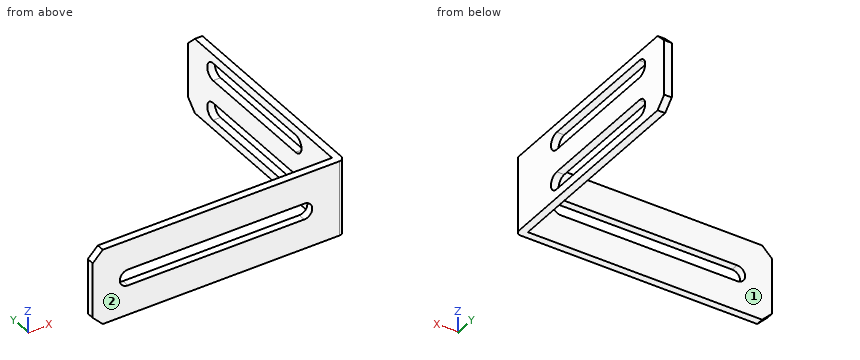
from build123d import *

# Parameters (mm, degrees)
BOSS_EXTRUDE1_DEPTH = 15
CUT_EXTRUDE1_DEPTH  = 2.5
CUT_EXTRUDE2_DEPTH  = 2.5
CHAMFER1_SIZE       = 2
FILLET1_R           = 1


with BuildPart() as part:
    # Sketch1 → Boss-Extrude1 (new body)
    with BuildSketch(Plane.XY):
        Polygon((-218.84057971, 0), (-170.34057971, 0), (-170.34057971, 43.5), (-168.84057971, 43.5), (-168.84057971, -1.5), (-218.84057971, -1.5), align=None)
    extrude(amount=BOSS_EXTRUDE1_DEPTH)

    # Sketch2 → Cut-Extrude1 (cut, through all)
    with BuildSketch(Plane(origin=(0, 0, 0), x_dir=(1, 0, 0), z_dir=(0, 1, 0))):
        with BuildLine():
            Line((-176.854809789, -9.1), (-211.854809789, -9.1))
            ThreePointArc((-211.854809789, -9.1), (-213.454809789, -7.5), (-211.854809789, -5.9))
            Line((-211.854809789, -5.9), (-176.854809789, -5.9))
            ThreePointArc((-176.854809789, -5.9), (-175.254809789, -7.5), (-176.854809789, -9.1))
        make_face()
    extrude(amount=-CUT_EXTRUDE1_DEPTH, mode=Mode.SUBTRACT)

    # Sketch3 → Cut-Extrude2 (cut, through all)
    with BuildSketch(Plane.ZY.offset(170.34057971)):
        with BuildLine():
            Line((1.75, 36), (1.75, 11))
            ThreePointArc((1.75, 11), (3.5, 9.25), (5.25, 11))
            Line((5.25, 11), (5.25, 36))
            ThreePointArc((5.25, 36), (3.5, 37.75), (1.75, 36))
        make_face()
        with BuildLine():
            Line((9.75, 36), (9.75, 11))
            ThreePointArc((9.75, 11), (11.5, 9.25), (13.25, 11))
            Line((13.25, 11), (13.25, 36))
            ThreePointArc((13.25, 36), (11.5, 37.75), (9.75, 36))
        make_face()
    extrude(amount=-CUT_EXTRUDE2_DEPTH, mode=Mode.SUBTRACT)

    # Chamfer1
    chamfer1_edges = [part.edges().sort_by_distance(p)[0] for p in [
        (-169.59057971, 43.5, 15),
        (-218.84057971, -0.75, 15),
        (-169.59057971, 43.5, 0),
        (-218.84057971, -0.75, 0),
    ]]
    chamfer(chamfer1_edges, length=CHAMFER1_SIZE)

    # Fillet1
    fillet1_edges = [part.edges().sort_by_distance(p)[0] for p in [
        (-168.84057971, -1.5, 7.5),
    ]]
    fillet(fillet1_edges, radius=FILLET1_R)


solid = part.part
Input: part model. Units: mm. Frame: model coordinates. Face numbers are marked on the shaded views. A direction names the side the tool comes from. Coordinates: 2 decimals unless noted, no trailing zeros. Loops run counter-clockwise (first coordinate to the right, second up) from the corner with the lowest first, then second, coordinate; pieces in that order, holes last. Notation, with made-up numbers: (10, 44.25) -> (18, 44.25) arc R13 ccw to (18, 63.25) -> close; hole circle Ø9 at (61, -21). An arc over 180 degrees is marked (long way). One line per item, written item: value.
(1) Cut plane B-B (z = 11.5). Output: boundary loops of the cut face in (x, y).
Answer below:
outline: (-218.84, -1.5) -> (-169.84, -1.5) arc R1 ccw to (-168.84, -0.5) -> (-168.84, 9.25) -> (-170.34, 9.25) -> (-170.34, 0) -> (-218.84, 0) -> close; (-170.34, 37.75) -> (-168.84, 37.75) -> (-168.84, 43.5) -> (-170.34, 43.5) -> close
(2) Cut plane A-A (x = -180). Output: boundary loops of the cut face in (y, z), then the cut area to 3 significant figures.
Answer below:
outline: (-1.5, 0) -> (0, 0) -> (0, 5.9) -> (-1.5, 5.9) -> close; (-1.5, 9.1) -> (0, 9.1) -> (0, 15) -> (-1.5, 15) -> close
area: 17.7 mm2
(3) Pin query (flat end, axial travel): pin 1 Ø4.5 at (y, z) = (13, 4) entering from -X. Return the tip coordinate at first contact, or that it passes through.
Answer below:
pin 1: stops at x = -170.34
(4) Cut plane D-D (z = 7.5). Output: boundary loops of the cut face in (x, y).
Answer below:
outline: (-218.84, -1.5) -> (-213.45, -1.5) -> (-213.45, 0) -> (-218.84, 0) -> close; (-175.25, -1.5) -> (-169.84, -1.5) arc R1 ccw to (-168.84, -0.5) -> (-168.84, 43.5) -> (-170.34, 43.5) -> (-170.34, 0) -> (-175.25, 0) -> close
(5) Set-up query: the marked faces 1 and 2. Return all of +Z, -Z, +X, -X, +Y, -Y with unobstructed straight access to the full face (end or side cutting, diameter ignored); none if empty.
Answer below:
face 1: +Z, -Z, -X, +Y
face 2: +Z, -Z, +X, -X, -Y
(6) Cut plane C-C (y = 30). Output: boundary loops of the cut face in (x, z).
Answer below:
outline: (-170.34, 0) -> (-168.84, 0) -> (-168.84, 1.75) -> (-170.34, 1.75) -> close; (-170.34, 5.25) -> (-168.84, 5.25) -> (-168.84, 9.75) -> (-170.34, 9.75) -> close; (-170.34, 13.25) -> (-168.84, 13.25) -> (-168.84, 15) -> (-170.34, 15) -> close
(7) Ray query, line 1 along X through (y, z) = (8, 5.75); line 2 along Y through (x, z) = (-198.5, 11). Return the intervals inside material, ascending.
Answer below:
line 1: x = -170.34 to -168.84
line 2: y = -1.5 to 0
